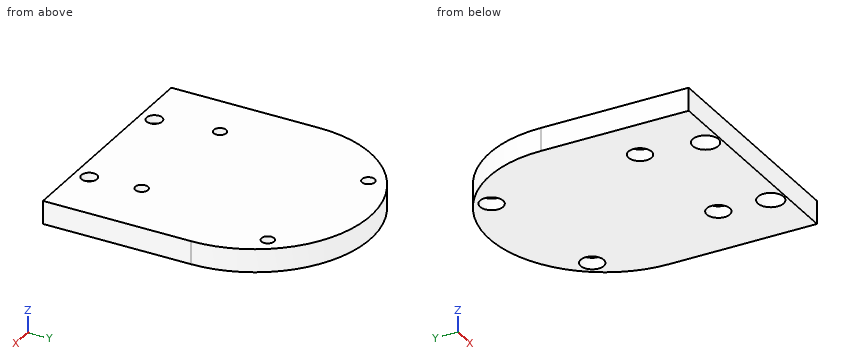
```python
from build123d import *

# Parameters (mm, degrees)
SKETCH1_R                                        = 50
SKETCH1_W                                        = 100
SKETCH1_H                                        = 64
BOSS_EXTRUDE1_DEPTH                              = 10
CBORE_FOR_M5_SHCS1_D                             = 5.5
CBORE_FOR_M5_SHCS1_CBORE_D                       = 10
CBORE_FOR_M5_SHCS1_CBORE_DEPTH                   = 5
CBORE_FOR_1_4_SOCKET_HEAD_CAP_SCREW1_D           = 6.7564
CBORE_FOR_1_4_SOCKET_HEAD_CAP_SCREW1_CBORE_D     = 11.1125
CBORE_FOR_1_4_SOCKET_HEAD_CAP_SCREW1_CBORE_DEPTH = 6.35


with BuildPart() as part:
    # Sketch1 → Boss-Extrude1 (new body)
    with BuildSketch(Plane.XY):
        Circle(SKETCH1_R)
        with Locations((0, -32)):
            Rectangle(SKETCH1_W, SKETCH1_H)
    extrude(amount=BOSS_EXTRUDE1_DEPTH)

    # CBORE for M5 SHCS1 (through all)
    with Locations(Plane(origin=(0, 0, 0), x_dir=(-1, 0, 0), z_dir=(0, 0, -1))):
        with Locations((-35.006967289, 24.970227096), (-23.419478506, -36.062834422), (29.325929483, -31.44820917), (23.419478506, 36.062834422)):
            CounterBoreHole(CBORE_FOR_M5_SHCS1_D / 2, CBORE_FOR_M5_SHCS1_CBORE_D / 2, CBORE_FOR_M5_SHCS1_CBORE_DEPTH)

    # CBORE for 1/4 Socket Head Cap Screw1 (through all)
    with Locations(Plane(origin=(0, 0, 0), x_dir=(-1, 0, 0), z_dir=(0, 0, -1))):
        with Locations((-25.4, -57.65), (25.4, -57.65)):
            CounterBoreHole(CBORE_FOR_1_4_SOCKET_HEAD_CAP_SCREW1_D / 2, CBORE_FOR_1_4_SOCKET_HEAD_CAP_SCREW1_CBORE_D / 2, CBORE_FOR_1_4_SOCKET_HEAD_CAP_SCREW1_CBORE_DEPTH)


solid = part.part
```
The listing builds one solid part. Answer for the finished solid, in the listing's coordinates (mm). Round coordinates to 2 decimals unless told otherwise and drop trailing zeros. Loops run counter-clockwise (first coordinate to the right, second up) from the corner with the lowest first, then second, coordinate; pieces in that order, holes last. Notation, with made-up numbers: (-25, 24) - (-6, 24) arc R6 ccw to (-6, 29) - close; hole circle Ø6 at (70, -19.5). An arc over 180 degrees is marked (long way). Return JSON: item names as keys, results as strings. Group by question number.
1. The part is cut by section C-C on x = -37. Determine the outline of the cut face in (y, z).
2. The part is cut by section A-A on z = 8.75. Determine the outline of the cut face in (x, y), then the cut area to 3 significant figures.
3. Consider probe 1 along X at (y, z) = (-36.5, 3.25); probe 2 along Y at (x, z) = (25.5, 4.75); probe 3 along Z at (x, y) = (25.5, -53.5). Determine where each line is inside the solid, lowest interval first.
4. The part is cut by section B-B on z = 2.75. Determine the outline of the cut face in (x, y).
5. Each of these flat-tipped pins is pushed along its axis until it touches: P1, Ø7, axis at x = -23.42, y = 36.06, coming from the -Z side; P2, Ø5, axis at y = 12.5, z = 8, coming from the -X side; P3, Ø11, axis at x = -25.4, y = -57.65, coming from the -Z side; P4, Ø4.5, axis at x = 23.42, y = -36.06, coming from the -Z side. Where does it stop, or does it pass through?
Resolved:
{
 "1": {"outline": "(-64, 0) - (33.63, 0) - (33.63, 10) - (-64, 10) - close"},
 "2": {"outline": "(-50, -64) - (50, -64) - (50, 0) arc R50 ccw to (-50, 0) - close; hole circle Ø5.5 at (-29.33, -31.45); hole circle Ø6.76 at (-25.4, -57.65); hole circle Ø5.5 at (-23.42, 36.06); hole circle Ø5.5 at (23.42, -36.06); hole circle Ø6.76 at (25.4, -57.65); hole circle Ø5.5 at (35.01, 24.97)", "area": "10,200 mm²"},
 "3": {"probe 1": "x = -50 to 18.44, 28.4 to 50", "probe 2": "y = -64 to -63.21, -52.09 to -40.61, -31.52 to 43.01", "probe 3": "z = 6.35 to 10"},
 "4": {"outline": "(-50, -64) - (50, -64) - (50, 0) arc R50 ccw to (-50, 0) - close; hole circle Ø10 at (-29.33, -31.45); hole circle Ø11.11 at (-25.4, -57.65); hole circle Ø10 at (-23.42, 36.06); hole circle Ø10 at (23.42, -36.06); hole circle Ø11.11 at (25.4, -57.65); hole circle Ø10 at (35.01, 24.97)"},
 "5": {"P1": "stops at z = 5", "P2": "stops at x = -48.99", "P3": "stops at z = 6.35", "P4": "passes through"}
}
